```python
from build123d import *

# Parameters (mm, degrees)
BOSS_EXTRUDE1_DEPTH = 10
SKETCH18_W          = 3.3
SKETCH18_H          = 2.5
CUT_EXTRUDE10_DEPTH = 43.3
SKETCH19_W          = 3.3
SKETCH19_H          = 2.5
CUT_EXTRUDE11_DEPTH = 43.3
SKETCH20_W          = 6.221233688
SKETCH20_H          = 2.5
CUT_EXTRUDE12_DEPTH = 57.710616844
SKETCH21_W          = 6.221233688
SKETCH21_H          = 2.5
CUT_EXTRUDE13_DEPTH = 57.710616844
SKETCH22_R          = 2.5
CUT_EXTRUDE14_DEPTH = 8.5
CUT_EXTRUDE15_DEPTH = 18.5
FILLET8_R           = 6


with BuildPart() as part:
    # Sketch1 → Boss-Extrude1 (new body)
    with BuildSketch(Plane(origin=(0, 0, 0), x_dir=(1, 0, 0), z_dir=(0, 1, 0))):
        Polygon((-21.15, 16.750923472), (-16.750923472, 21.15), (16.750923472, 21.15), (21.15, 16.750923472), (21.15, -16.750923472), (16.750923472, -21.15), (-16.750923472, -21.15), (-21.15, -16.750923472), align=None)
    boss_extrude1 = extrude(amount=BOSS_EXTRUDE1_DEPTH)

    # Sketch18 → Cut-Extrude10 (cut, through all)
    with BuildSketch(Plane.XY.offset(21.15)):
        with Locations((15.100923472, 8.75)):
            Rectangle(SKETCH18_W, SKETCH18_H)
        with Locations((-15.100923472, 8.75)):
            Rectangle(SKETCH18_W, SKETCH18_H)
    cut_extrude10 = extrude(amount=-CUT_EXTRUDE10_DEPTH, mode=Mode.SUBTRACT)

    # Sketch19 → Cut-Extrude11 (cut, through all)
    with BuildSketch(Plane(origin=(21.15, 0, 0), x_dir=(0, 0, -1), z_dir=(1, 0, 0))):
        with Locations((-15.100923472, 8.75)):
            Rectangle(SKETCH19_W, SKETCH19_H)
        with Locations((15.100923472, 8.75)):
            Rectangle(SKETCH19_W, SKETCH19_H)
    cut_extrude11 = extrude(amount=-CUT_EXTRUDE11_DEPTH, mode=Mode.SUBTRACT)

    # Sketch20 → Cut-Extrude12 (cut, through all)
    with BuildSketch(Plane(origin=(18.950461736, 0, 18.950461736), x_dir=(0.707106781, 0, -0.707106781), z_dir=(0.707106781, 0, 0.707106781))):
        with Locations((0, 8.75)):
            Rectangle(SKETCH20_W, SKETCH20_H)
    cut_extrude12 = extrude(amount=-CUT_EXTRUDE12_DEPTH, mode=Mode.SUBTRACT)

    # Sketch21 → Cut-Extrude13 (cut, through all)
    with BuildSketch(Plane(origin=(-18.950461736, 0, 18.950461736), x_dir=(0.707106781, 0, 0.707106781), z_dir=(-0.707106781, 0, 0.707106781))):
        with Locations((0, 8.75)):
            Rectangle(SKETCH21_W, SKETCH21_H)
    cut_extrude13 = extrude(amount=-CUT_EXTRUDE13_DEPTH, mode=Mode.SUBTRACT)

    # Sketch22 → Cut-Extrude14 (cut, through all)
    with BuildSketch(Plane(origin=(0, 7.5, 0), x_dir=(1, 0, 0), z_dir=(0, 1, 0))):
        Circle(SKETCH22_R)
    cut_extrude14 = extrude(amount=-CUT_EXTRUDE14_DEPTH, mode=Mode.SUBTRACT)

    # Mirror1: Boss-Extrude1, Cut-Extrude10, Cut-Extrude11, Cut-Extrude12, Cut-Extrude13, Cut-Extrude14 across plane
    add(boss_extrude1.mirror(Plane(origin=(0, 0, 0), x_dir=(0, 0, 1), z_dir=(0, -1, 0))))
    add(cut_extrude10.mirror(Plane(origin=(0, 0, 0), x_dir=(0, 0, 1), z_dir=(0, -1, 0))), mode=Mode.SUBTRACT)
    add(cut_extrude11.mirror(Plane(origin=(0, 0, 0), x_dir=(0, 0, 1), z_dir=(0, -1, 0))), mode=Mode.SUBTRACT)
    add(cut_extrude12.mirror(Plane(origin=(0, 0, 0), x_dir=(0, 0, 1), z_dir=(0, -1, 0))), mode=Mode.SUBTRACT)
    add(cut_extrude13.mirror(Plane(origin=(0, 0, 0), x_dir=(0, 0, 1), z_dir=(0, -1, 0))), mode=Mode.SUBTRACT)
    add(cut_extrude14.mirror(Plane(origin=(0, 0, 0), x_dir=(0, 0, 1), z_dir=(0, -1, 0))), mode=Mode.SUBTRACT)

    # Sketch23 → Cut-Extrude15 (cut, through all)
    with BuildSketch(Plane(origin=(0, 7.5, 0), x_dir=(1, 0, 0), z_dir=(0, 1, 0))):
        Polygon((-21.15, -14.432485579), (-14.432485579, -21.15), (-16.750923472, -21.15), (-21.15, -16.750923472), align=None)
        Polygon((-21.15, 14.432485579), (-14.432485579, 21.15), (-16.750923472, 21.15), (-21.15, 16.750923472), align=None)
        Polygon((14.432485579, 21.15), (21.15, 14.432485579), (21.15, 16.750923472), (16.750923472, 21.15), align=None)
        Polygon((14.432485579, -21.15), (21.15, -14.432485579), (21.15, -16.750923472), (16.750923472, -21.15), align=None)
    extrude(amount=-CUT_EXTRUDE15_DEPTH, mode=Mode.SUBTRACT)

    # Fillet8
    fillet8_edges = [part.edges().sort_by_distance(p)[0] for p in [
        (14.432485579, 0, -21.15),
        (21.15, 0, -14.432485579),
        (-21.15, 0, -14.432485579),
        (-14.432485579, 0, -21.15),
        (-14.432485579, 0, 21.15),
        (-21.15, 0, 14.432485579),
        (21.15, 0, 14.432485579),
        (14.432485579, 0, 21.15),
    ]]
    fillet(fillet8_edges, radius=FILLET8_R)


solid = part.part
```
Input: part model. Units: mm. Frame: model coordinates. A direction names the side the tool comes from. Coordinates: 2 decimals unless noted, no trailing zeros. Loops run counter-clockwise (first coordinate to the right, second up) from the corner with the lowest first, then second, coordinate; pieces in that order, holes last. Notation, with made-up numbers: M 70,55.25 L 87,55.25 A28 ccw 87,74.25 Z; hole C -23,53 d2. An arc over 180 degrees is marked long. Answer in a Markdown table with one row per item.
1. Section A-A, the plane y = -2.75. Output: boundary loops of the cut face in (x, z).
Response:
| item | result |
|---|---|
| outline | M -21.15,-11.95 A6 ccw -19.39,-16.19 L -16.19,-19.39 A6 ccw -11.95,-21.15 L 11.95,-21.15 A6 ccw 16.19,-19.39 L 19.39,-16.19 A6 ccw 21.15,-11.95 L 21.15,11.95 A6 ccw 19.39,16.19 L 16.19,19.39 A6 ccw 11.95,21.15 L -11.95,21.15 A6 ccw -16.19,19.39 L -19.39,16.19 A6 ccw -21.15,11.95 Z; hole C 0,0 d5 |
2. Material intervals for line 1 (X direction, y = 4.25, z = 0); line 2 (Z direction, x = -8, y = -8.75), sorted ascending.
Response:
| item | result |
|---|---|
| line 1 | x = -21.15 to -2.5, 2.5 to 21.15 |
| line 2 | z = -21.15 to -16.75, -13.45 to -12.4, -3.6 to 3.6, 12.4 to 13.45, 16.75 to 21.15 |
3. Section C-C, the plane z = -3.5. Output: boundary loops of the cut face in (x, y), then the cut area to 3 significant figures.
Response:
| item | result |
|---|---|
| outline | M -21.15,-10 L -16.75,-10 L -16.75,-7.5 L -13.45,-7.5 L -13.45,-10 L -7.9,-10 L -7.9,-7.5 L 7.9,-7.5 L 7.9,-10 L 13.45,-10 L 13.45,-7.5 L 16.75,-7.5 L 16.75,-10 L 21.15,-10 L 21.15,10 L 16.75,10 L 16.75,7.5 L 13.45,7.5 L 13.45,10 L 7.9,10 L 7.9,7.5 L -7.9,7.5 L -7.9,10 L -13.45,10 L -13.45,7.5 L -16.75,7.5 L -16.75,10 L -21.15,10 Z |
| area | 734 mm2 |
4. First-contact query: pin 1 (0.8 mm diameter, centred on x = 19.5, y = 8.5, fed in from +Z); pin 2 (5 mm diameter, centred on x = 15, y = -5, fed in from -Z); pin 3 (8 mm diameter, centred on x = 0, z = 0, fed in from -Y). Flat tips, straight axial feed; report the tip coordinate or a pass-through.
Response:
| item | result |
|---|---|
| pin 1 | stops at z = 13.45 |
| pin 2 | stops at z = -21.12 |
| pin 3 | stops at y = -7.5 |
5. Section D-D, the plane x = 14.5. Output: boundary loops of the cut face in (y, z), then the cut area to 3 significant figures.
Response:
| item | result |
|---|---|
| outline | M -7.5,-20.58 L 7.5,-20.58 L 7.5,20.58 L -7.5,20.58 Z |
| area | 617 mm2 |
6. Reachability of faces 1 (the flat face through (13.451, -9, -19)), 2 (the flat face through (0, -9, -13.451)), 3 (the flat face through (-8.9, -8.7, -4.5)), 4 (the flat face through (12.9, 8.7, 17.3)), 5 (the flat face through (12.9, -8.7, -17.3)) from +Z, -Z, +X, -X, +Y, -Y: full face, straight path, thin tool, end or side. Return the list, or none.
Response:
| item | result |
|---|---|
| face 1 | +Z, -Z, +X, -Y |
| face 2 | +X, -X, -Y |
| face 3 | -Y |
| face 4 | +X, +Y |
| face 5 | +X, -Y |
